Here's how the part is built. I have some questions about the finished solid (model axes, mm). A direction names the side the tool comes from. Coordinates: 2 decimals unless noted, no trailing zeros. Answer as CSV lines item,"result". Start each with the question number.
Item 1: We'd pull the mould along X, two halves only. Please class faces 1 (the face through (0, 15, -99)), 2 (the face through (0.8, 9.7, -192.4)): pulls with the +X half, pulls with the -X half, needs draft (parallel to the pull), parting line crosses it, or undercut.
Item 2: I'm going to push flat-ended pins straight in: pin 1 (1.5 mm diameter, centred on y = 9, z = -94, fed in from -X); pin 2 (2.5 mm diameter, centred on y = 8, z = -66.5, fed in from +X); pin 3 (1.7 mm diameter, centred on y = 7, z = -110.5, fed in from -X). Where does each tip first touch, or does it pass through?
Item 3: I need wall thicknesses on line 1 (Z direction, x = 0, y = 10.75); line 2 (Z direction, x = 0, y = 6.5); line 3 (X direction, y = 13.2, z = -130). Which ranges of each line are inside material? Lowest first, please.
Item 4: On a 3-axis mill with a long thin cutter (end or side, diameter ignored), from which of +Z, -Z, +X, -X, +Y, -Y can I reach the whole of each face in a straight line? I mean faces 3 (the face through (0, 0, -99)), 4 (the face through (1.436, 12.386, -186.536)). Say none if no direction works.
Item 5: Imagine slicing it at A-A on x = 0. Count the separate pieces of the cut face and the enclosed holes in it, and give its area (3 significant figures).
from build123d import *

# Parameters (mm, degrees)
BODY_DEPTH                                 = 200
AESTHETIC_CHAMFER_SIZE                     = 0.15
PRODUCTION_FILLET_R                        = 0.1
MOUNTING_HOLES_PATTERN_COUNT               = 4
MOUNTING_HOLES_PATTERN_PITCH               = 60
PRODUCTION_FILLET_OF_MOUNTING_HOLES_PATT_R = 0.1


with BuildPart() as part:
    # Rail Profile → Body (new body)
    with BuildSketch(Plane.XY):
        with BuildLine():
            Line((-7, 0), (7, 0))
            Line((7, 0), (7.5, 0.5))
            Line((7.5, 0.5), (7.5, 3.085786438))
            ThreePointArc((7.5, 3.085786438), (7.423879533, 3.46846987), (7.207106781, 3.792893219))
            Line((7.207106781, 3.792893219), (4.867157288, 6.132842712))
            ThreePointArc((4.867157288, 6.132842712), (4.780448187, 6.262612052), (4.75, 6.415685425))
            Line((4.75, 6.415685425), (4.75, 8.584314575))
            ThreePointArc((4.75, 8.584314575), (4.780448187, 8.737387948), (4.867157288, 8.867157288))
            Line((4.867157288, 8.867157288), (5.062965362, 9.062965362))
            ThreePointArc((5.062965362, 9.062965362), (5.134996734, 9.161242682), (5.17409812, 9.27664646))
            ThreePointArc((5.17409812, 9.27664646), (5.61862915, 10.13137085), (6.47335354, 10.57590188))
            ThreePointArc((6.47335354, 10.57590188), (6.694124352, 10.694306692), (6.801170165, 10.920803148))
            ThreePointArc((6.801170165, 10.920803148), (6.915305692, 11.154571658), (7.149074202, 11.268707185))
            ThreePointArc((7.149074202, 11.268707185), (7.399691242, 11.400760606), (7.5, 11.665685425))
            Line((7.5, 11.665685425), (7.5, 12.334314575))
            ThreePointArc((7.5, 12.334314575), (7.399691242, 12.599239394), (7.149074202, 12.731292815))
            ThreePointArc((7.149074202, 12.731292815), (6.915305692, 12.845428342), (6.801170165, 13.079196852))
            ThreePointArc((6.801170165, 13.079196852), (6.694124352, 13.305693308), (6.47335354, 13.42409812))
            ThreePointArc((6.47335354, 13.42409812), (5.61862915, 13.86862915), (5.17409812, 14.72335354))
            ThreePointArc((5.17409812, 14.72335354), (5.134996734, 14.838757318), (5.062965362, 14.937034638))
            Line((5.062965362, 14.937034638), (5, 15))
            Line((5, 15), (-5, 15))
            Line((-5, 15), (-5.062965362, 14.937034638))
            ThreePointArc((-5.062965362, 14.937034638), (-5.134996734, 14.838757318), (-5.17409812, 14.72335354))
            ThreePointArc((-5.17409812, 14.72335354), (-5.61862915, 13.86862915), (-6.47335354, 13.42409812))
            ThreePointArc((-6.47335354, 13.42409812), (-6.694124352, 13.305693308), (-6.801170165, 13.079196852))
            ThreePointArc((-6.801170165, 13.079196852), (-6.915305692, 12.845428342), (-7.149074202, 12.731292815))
            ThreePointArc((-7.149074202, 12.731292815), (-7.399691242, 12.599239394), (-7.5, 12.334314575))
            Line((-7.5, 12.334314575), (-7.5, 11.665685425))
            ThreePointArc((-7.5, 11.665685425), (-7.399691242, 11.400760606), (-7.149074202, 11.268707185))
            ThreePointArc((-7.149074202, 11.268707185), (-6.915305692, 11.154571658), (-6.801170165, 10.920803148))
            ThreePointArc((-6.801170165, 10.920803148), (-6.694124352, 10.694306692), (-6.47335354, 10.57590188))
            ThreePointArc((-6.47335354, 10.57590188), (-5.61862915, 10.13137085), (-5.17409812, 9.27664646))
            ThreePointArc((-5.17409812, 9.27664646), (-5.134996734, 9.161242682), (-5.062965362, 9.062965362))
            Line((-5.062965362, 9.062965362), (-4.867157288, 8.867157288))
            ThreePointArc((-4.867157288, 8.867157288), (-4.780448187, 8.737387948), (-4.75, 8.584314575))
            Line((-4.75, 8.584314575), (-4.75, 6.415685425))
            ThreePointArc((-4.75, 6.415685425), (-4.780448187, 6.262612052), (-4.867157288, 6.132842712))
            Line((-4.867157288, 6.132842712), (-7.207106781, 3.792893219))
            ThreePointArc((-7.207106781, 3.792893219), (-7.423879533, 3.46846987), (-7.5, 3.085786438))
            Line((-7.5, 3.085786438), (-7.5, 0.5))
            Line((-7.5, 0.5), (-7, 0))
        make_face()
    extrude(amount=-BODY_DEPTH)

    # Aesthetic Chamfer
    aesthetic_chamfer_edges = [part.edges().sort_by_distance(p)[0] for p in [
        (7.423879533, 3.46846987, -200),
        (-5.134996734, 9.161242682, -200),
        (-4.965061325, 8.965061325, -200),
        (-4.780448187, 8.737387948, -200),
        (-4.75, 7.5, -200),
        (-4.780448187, 6.262612052, -200),
        (-6.037132034, 4.962867966, -200),
        (-7.423879533, 3.46846987, -200),
        (-7.5, 1.792893219, -200),
        (-7.25, 0.25, -200),
        (0, 0, -200),
        (6.037132034, 4.962867966, -200),
        (4.780448187, 6.262612052, -200),
        (4.75, 7.5, -200),
        (4.780448187, 8.737387948, -200),
        (4.965061325, 8.965061325, -200),
        (5.134996734, 9.161242682, -200),
        (5.61862915, 10.13137085, -200),
        (6.694124352, 10.694306692, -200),
        (0, 0, 0),
        (-7.25, 0.25, 0),
        (-7.5, 1.792893219, 0),
        (-7.423879533, 3.46846987, 0),
        (-6.037132034, 4.962867966, 0),
        (-4.780448187, 6.262612052, 0),
        (6.915305692, 11.154571658, -200),
        (-4.75, 7.5, 0),
        (-4.780448187, 8.737387948, 0),
        (-4.965061325, 8.965061325, 0),
        (-5.134996734, 9.161242682, 0),
        (-5.61862915, 10.13137085, 0),
        (-6.694124352, 10.694306692, 0),
        (-6.915305692, 11.154571658, 0),
        (7.25, 0.25, -200),
        (7.399691242, 11.400760606, -200),
        (-7.399691242, 11.400760606, 0),
        (-7.5, 12, 0),
        (-7.399691242, 12.599239394, 0),
        (-6.915305692, 12.845428342, 0),
        (-6.694124352, 13.305693308, 0),
        (-5.61862915, 13.86862915, 0),
        (-5.134996734, 14.838757318, 0),
        (-5.031482681, 14.968517319, 0),
        (7.5, 12, -200),
        (0, 15, 0),
        (5.031482681, 14.968517319, 0),
        (5.134996734, 14.838757318, 0),
        (5.61862915, 13.86862915, 0),
        (6.694124352, 13.305693308, 0),
        (6.915305692, 12.845428342, 0),
        (7.399691242, 12.599239394, 0),
        (7.399691242, 12.599239394, -200),
        (7.5, 12, 0),
        (7.399691242, 11.400760606, 0),
        (6.915305692, 11.154571658, 0),
        (6.694124352, 10.694306692, 0),
        (5.61862915, 10.13137085, 0),
        (5.134996734, 9.161242682, 0),
        (4.965061325, 8.965061325, 0),
        (4.780448187, 8.737387948, 0),
        (6.915305692, 12.845428342, -200),
        (4.75, 7.5, 0),
        (4.780448187, 6.262612052, 0),
        (6.037132034, 4.962867966, 0),
        (7.423879533, 3.46846987, 0),
        (7.5, 1.792893219, 0),
        (7.25, 0.25, 0),
        (6.694124352, 13.305693308, -200),
        (5.61862915, 13.86862915, -200),
        (5.134996734, 14.838757318, -200),
        (5.031482681, 14.968517319, -200),
        (0, 15, -200),
        (-5.031482681, 14.968517319, -200),
        (7.5, 1.792893219, -200),
        (-5.134996734, 14.838757318, -200),
        (-5.61862915, 13.86862915, -200),
        (-6.694124352, 13.305693308, -200),
        (-6.915305692, 12.845428342, -200),
        (-7.399691242, 12.599239394, -200),
        (-7.5, 12, -200),
        (-7.399691242, 11.400760606, -200),
        (-6.915305692, 11.154571658, -200),
        (-6.694124352, 10.694306692, -200),
        (-5.61862915, 10.13137085, -200),
    ]]
    chamfer(aesthetic_chamfer_edges, length=AESTHETIC_CHAMFER_SIZE)

    # Sketch1 → Mounting Hole (revolve, cut)
    with BuildSketch(Plane(origin=(0, 15, -10), x_dir=(0, 0, 1), z_dir=(1, 0, 0))):
        Polygon((0, 0), (0, 15), (2.35, 15), (2.25, 14.9), (2.25, 5.4), (2.35, 5.3), (3.75, 5.3), (3.75, 0.1), (3.85, 0), align=None)
    mounting_hole = revolve(axis=Axis((0, 21.35, -10), (0, -1, 0)), mode=Mode.SUBTRACT)

    # Production Fillet
    production_fillet_edges = [part.edges().sort_by_distance(p)[0] for p in [
        (0, 9.7, -13.75),
    ]]
    fillet(production_fillet_edges, radius=PRODUCTION_FILLET_R)

    # Mounting Holes Pattern: Mounting Hole ×4
    with Locations(*[(0, 0, -i * MOUNTING_HOLES_PATTERN_PITCH) for i in range(1, MOUNTING_HOLES_PATTERN_COUNT)]):
        add(mounting_hole, mode=Mode.SUBTRACT)

    # Production Fillet of Mounting Holes Patt
    production_fillet_of_mounting_holes_patt_edges = [part.edges().sort_by_distance(p)[0] for p in [
        (0, 9.7, -73.75),
        (0, 9.7, -133.75),
        (0, 9.7, -193.75),
    ]]
    fillet(production_fillet_of_mounting_holes_patt_edges, radius=PRODUCTION_FILLET_OF_MOUNTING_HOLES_PATT_R)


solid = part.part
Responses:
1,face 1,"needs draft"
1,face 2,"undercut"
2,pin 1,"stops at x = -5.34"
2,pin 2,"stops at x = 5.17"
2,pin 3,"stops at x = -4.85"
3,line 1,"z = -200 to -193.75, -186.25 to -133.75, -126.25 to -73.75, -66.25 to -13.75, -6.25 to 0"
3,line 2,"z = -200 to -192.25, -187.75 to -132.25, -127.75 to -72.25, -67.75 to -12.25, -7.75 to 0"
3,line 3,"x = -6.77 to -3.75, 3.75 to 6.77"
4,face 3,"+Z, -Z, +X, -X, -Y"
4,face 4,"+Y"
5,separate pieces,"5"
5,enclosed holes,"0"
5,area,"2,670 mm^2"
